from build123d import *

# Parameters (mm, degrees)
CYLINDER083_R          = 2.75
CYLINDER083_DEPTH      = 7
CYLINDER082_R          = 4
CYLINDER082_DEPTH      = 9
CYLINDER070_R          = 1.38
CYLINDER070_DEPTH      = 10
CYLINDER072_R          = 2.25
CYLINDER072_DEPTH      = 10
BOX040_W               = 25
BOX040_H               = 10
BOX040_DEPTH           = 4
CUT048_PLACEMENT_ANGLE = 30
FILLET007_R            = 3


with BuildPart() as cilindro003:
    # Cylinder083 → Cylinder083 (new body)
    with BuildSketch(Plane(origin=(17, 17, 12), x_dir=(1, 0, 0), z_dir=(0, 0, 1))):
        Circle(CYLINDER083_R)
    extrude(amount=CYLINDER083_DEPTH)


with BuildPart() as obj1:
    # Cylinder082 → Cylinder082 (new body)
    with BuildSketch(Plane(origin=(17, 17, 10), x_dir=(1, 0, 0), z_dir=(0, 0, 1))):
        Circle(CYLINDER082_R)
    extrude(amount=CYLINDER082_DEPTH)

    # Cut054: cut Cilindro003
    add(cilindro003.part, mode=Mode.SUBTRACT)


with BuildPart() as obj1_1:
    # Cut054 placement: moved
    add(obj1.part.moved(Location((21, 102, 52))))


with BuildPart() as cylinder070:
    # Cylinder070 → Cylinder070 (new body)
    with BuildSketch(Plane(origin=(25, 52, 59), x_dir=(1, 0, 0), z_dir=(0, 0, 1))):
        Circle(CYLINDER070_R)
    extrude(amount=CYLINDER070_DEPTH)


with BuildPart() as cylinder072:
    # Cylinder072 → Cylinder072 (new body)
    with BuildSketch(Plane(origin=(40, 52, 59), x_dir=(1, 0, 0), z_dir=(0, 0, 1))):
        Circle(CYLINDER072_R)
    extrude(amount=CYLINDER072_DEPTH)


with BuildPart() as fusion010:
    # Box040 → Box040 (new body)
    with BuildSketch(Plane(origin=(45, 57, 62), x_dir=(-1, 0, 0), z_dir=(0, 0, 1))):
        with Locations((12.5, 5)):
            Rectangle(BOX040_W, BOX040_H)
    extrude(amount=BOX040_DEPTH)

    # Cut047: cut Cylinder072
    add(cylinder072.part, mode=Mode.SUBTRACT)

    # Cut048: cut Cylinder070
    add(cylinder070.part, mode=Mode.SUBTRACT)


with BuildPart() as fusion010_1:
    # Cut048 placement: moved
    add(fusion010.part.moved(Location((31.35, -13.05, 0))).rotate(Axis((31.35, -13.05, 0), (0, 0, 1)), CUT048_PLACEMENT_ANGLE))

    # Fillet007
    fillet007_edges = [fusion010_1.edges().sort_by_distance(p)[0] for p in [
        (20.170508, 46.313448, 64),
        (25.170508, 37.653194, 64),
    ]]
    fillet(fillet007_edges, radius=FILLET007_R)


with BuildPart() as fusion010_2:
    # Fillet007 placement: moved
    add(fusion010_1.part.moved(Location((-2, 67, 0))))

    # Fusion010: union obj1
    add(obj1_1.part)


solid = fusion010_2.part
For this review, take the finished solid that the model builds, in its own axes (mm). A direction names the side the tool comes from. Round coordinates to 2 decimals unless told otherwise and drop trailing zeros. Order: outer loops, then holes, each group sorted by start corner. A loop starts at its lowest first (then second) coordinate and runs counter-clockwise, first axis right, second up. Notation, with made-up numbers: M 13.25,79 L 56.25,79 A7 ccw 56.25,83 Z; hole C 65,80 d11. An arc over 180 degrees is marked long. Use a Markdown table: item, result. Add a question column.
Item 1: Add section C-C, the plane z = 70. Give the boundary of the cut face in (x, y), then the cut area to 3 significant figures.
Item 2: Add section A-A, the plane z = 65.5. Give the boundary of the cut face in (x, y).
Item 3: Insertion check: pin 1 (5 mm diameter, centred on x = 42, z = 68.5, fed in from +Y); pin 2 (3.5 mm diameter, centred on x = 37.99, y = 118.98, fed in from +Z); pin 3 (5 mm diameter, centred on x = 27, y = 113.5, fed in from +Z); pin 4 (2.5 mm diameter, centred on x = 25, y = 111.48, fed in from +Z). Each pin has a flat end and moves straight along its axis. Give the tip position at first contact, or say it passes through.
Item 4: To check wall thickness, follow line 1 along X through (y, z) = (119, 69.5); line 2 along Z through (x, y) = (34, 117.25); line 3 along X through (y, z) = (117.25, 65.5). State the ranges of each line that lie inside material, in increasing order.
Item 5: Tool access review of faces 1 (the flat face through (37, 116, 71)), 2 (the cylindrical face through (35.818, 117.327, 68.465)): name each direction out of +Z, -Z, +X, -X, +Y, -Y from which nothing blocks a thin tool from reaching the whole face with its end or side.
Item 6: Add section D-D, the plane y = 119. Give the boundary of the cut face in (x, z), then the cut area to 3 significant figures.
Item 7: Mouldability with a two-part tool opening along X and no side actions: class faces 3 (the cylindrical face through (23.653, 111.782, 63.972)), 4 (the cylindrical face through (40.22, 119.28, 64.99)), 5 (the cylindrical face through (37.479, 122.966, 68.465)), 6 (the cylindrical face through (19.38, 113.02, 64.03)) as released by +X, released by -X, zero draft, split by the parting line, or undercut.
Item 8: Add section B-B, the plane x = 38. Give the boundary of the cut face in (y, z) (3 decimals).
Geometry results:
| question | item | result |
|---|---|---|
| 1 | outline | C 38,119 d8; hole C 38,119 d5.5 |
| 1 | area | 26.5 mm² |
| 2 | outline | M 19.67,110.72 L 21.67,107.25 A3 ccw 25.77,106.15 L 44.82,117.15 L 39.82,125.81 L 20.77,114.81 A3 ccw Z; hole C 25,111.48 d2.76; hole C 37.99,118.98 d4.5 |
| 3 | pin 1 | stops at y = 122.71 |
| 3 | pin 2 | stops at z = 64 |
| 3 | pin 3 | stops at z = 66 |
| 3 | pin 4 | passes through |
| 4 | line 1 | x = 34 to 35.25, 40.75 to 42 |
| 4 | line 2 | z = 62 to 66 |
| 4 | line 3 | x = 24.99 to 36.56, 39.43 to 44.77 |
| 5 | face 1 | +Z, +X, -X, +Y, -Y |
| 5 | face 2 | +Z |
| 6 | outline | M 28.02,62 L 43.75,62 L 43.75,66 L 42,66 L 42,71 L 40.75,71 L 40.75,66 L 40.24,66 L 40.24,64 L 35.74,64 L 35.74,66 L 35.25,66 L 35.25,71 L 34,71 L 34,66 L 28.02,66 Z |
| 6 | area | 66.4 mm² |
| 7 | face 3 | undercut |
| 7 | face 4 | undercut |
| 7 | face 5 | split by the parting line |
| 7 | face 6 | released by -X |
| 8 | outline | M 113.215,62 L 124.762,62 L 124.762,66 L 123,66 L 123,71 L 121.75,71 L 121.75,66 L 121.233,66 L 121.233,64 L 116.733,64 L 116.733,66 L 116.25,66 L 116.25,71 L 115,71 L 115,66 L 113.215,66 Z |
